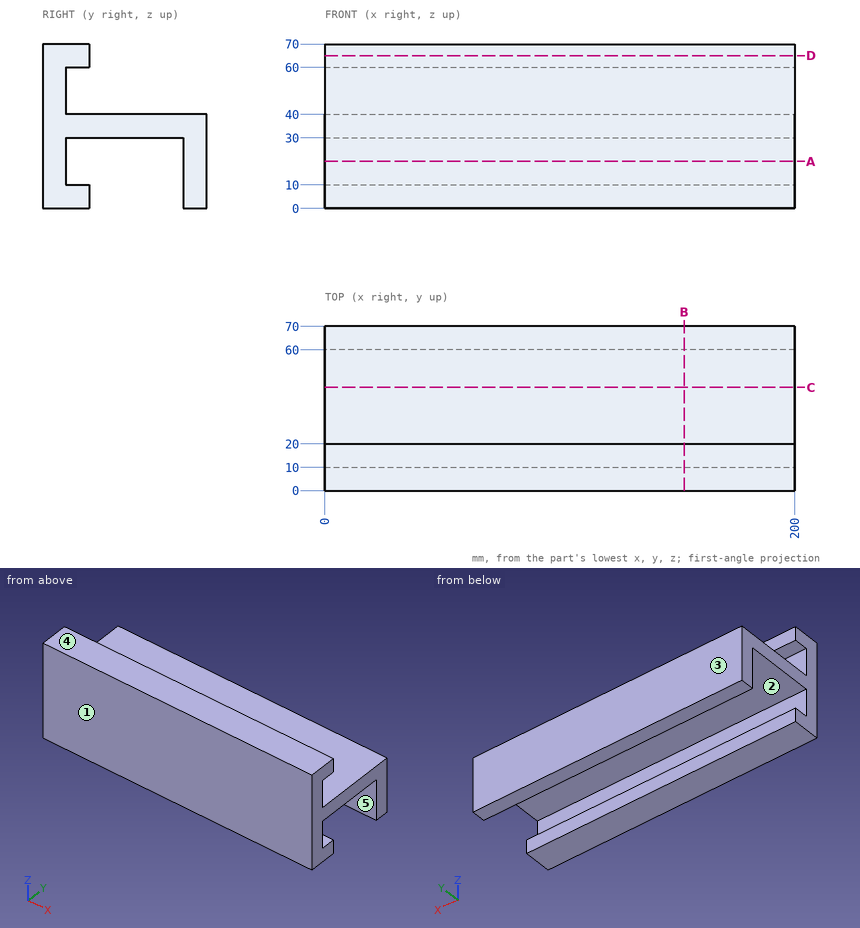
Check sheet for the drawn part. Datum: minimum x, y, z corner. Units: mm. A direction names the side the tool comes from. Round coordinates to 2 decimals unless told otherwise and drop trailing zeros. Loops run counter-clockwise (first coordinate to the right, second up) from the corner with the lowest first, then second, coordinate; pieces in that order, holes last. Notation, with made-up numbers: M -33,17.25 L 8,17.25 A19 ccw 8,29.25 Z; hole C 80.5,4.5 d11. An arc over 180 degrees is marked long. One line per question, with ' | ' between items. Start each with the question number.
Item 1: Section check C-C (y = 44). Record the boundary of the cut face in (x, z).
Item 2: Set-up check for the marked faces 4 and 5: record each of +Z, -Z, +X, -X, +Y, -Y from which the full face is reachable in a straight line by a thin tool's end or side.
Item 3: Release check for a two-part mould opening along Y. For the marked faces 1, 2 and 3 record: released by +Y, released by -Y, zero draft, split by the parting line, or undercut.
Item 4: Section check D-D (z = 65). Record the boundary of the cut face in (x, y).
Item 5: Section check A-A (z = 20). Record the boundary of the cut face in (x, y).
Item 6: Section check B-B (x = 153). Record the boundary of the cut face in (y, z).
Item 7: Scan lines: probe 1 along Z at (x, y) = (143.5, 15); probe 2 along Y at (x, z) = (120, 24); probe 3 along Y at (x, z) = (162.5, 42). Record each from-to range of solid material in increasing order.
Item 8: Gauge pin test, flat ends, axial feed: pin 1 Ø4 at (x, y) = (123.5, 61.5) entering from +Z; pin 2 Ø12 at (x, z) = (176, 60) entering from +Y; pin 3 Ø16 at (x, z) = (138.5, 51) entering from +Y. Record the tip position at first contact, or that the pin passes through.
Worked out:
1) outline: M 0,30 L 200,30 L 200,40 L 0,40 Z
2) face 4: +Z, +X, -X, +Y, -Y | face 5: -Z, +X, -X
3) face 1: released by -Y | face 2: undercut | face 3: released by +Y
4) outline: M 0,0 L 200,0 L 200,20 L 0,20 Z
5) outline: M 0,0 L 200,0 L 200,10 L 0,10 Z; M 0,60 L 200,60 L 200,70 L 0,70 Z
6) outline: M 0,0 L 20,0 L 20,10 L 10,10 L 10,30 L 60,30 L 60,0 L 70,0 L 70,40 L 10,40 L 10,60 L 20,60 L 20,70 L 0,70 Z
7) probe 1: 0 to 10, 30 to 40, 60 to 70 | probe 2: 0 to 10, 60 to 70 | probe 3: 0 to 10
8) pin 1: z = 40 | pin 2: y = 20 | pin 3: y = 10
